Source: CAD feature listing. Evaluate the final solid. Frame: model axes, mm. A direction names the side the tool comes from. Give positions to 0.01 mm unless a question says otherwise; leave off trailing zeros. Write each loop counter-clockwise with the first axis right and the second up, starting at its lowest first coordinate (ties: lowest second). Pieces come first, ordered by that corner, then holes. Notation, with made-up numbers: (-5, 36) -> (27, 36) arc R19 ccw to (27, 69) -> close; hole circle Ø7 at (0.25, -13.5). An arc over 180 degrees is marked (long way). Answer as a JSON object with one key per item and string values. Group by question number.
Item 1: Pull-direction query (Y, two-part tool) for faces 4 (the face through (2, -1, 46.038)), 5 (the face through (2, 69.85, 25)), 6 (the face through (-127, -0.3, 27.4)); classes: pulls with the +Y half, pulls with the -Y half, needs draft (parallel to the pull), parting line crosses it, or undercut.
Item 2: Section query C-C on x = 106.5. Return the cut outline in (y, z), plus the area to 3 significant figures.
Item 3: Section query B-B on y = 11. Return the cut outline in (x, z), plus the area to 3 significant figures.
Item 4: Access query for faces 1 (the face through (2, 35, 0)), 2 (the face through (2, 0.127, 23)), 3 (the face through (2, 35, 4.762)). Directions: +Z, -Z, +X, -X, +Y, -Y. A direction counts if a zero-diameter tool reaches every point of the face in a straight line with its end or side. Return the directions, or none.
Item 5: Section query A-A on z = 9. Return the cut outline in (x, y).
Item 6: Ray query, probe 1 along Y at (x, z) = (20, 33); probe 2 along Z at (x, y) = (-25, 44); probe 3 along Y at (x, z) = (-112, 46). Return the intervals inside material, ascending. Write a range as from..to.
from build123d import *

# Parameters (mm, degrees)
F1_DEPTH = 127


with BuildPart() as f1:
    # F0 (on Right) → F1 (new body, symmetric)
    with BuildSketch(Plane.YZ):
        Polygon((69.85, 50.8), (-69.85, 50.8), (-69.85, 0), (-0.127, 0), (-0.127, 45.7835), (-4.7625, 45.7835), (-4.7625, 4.7625), (-65.0875, 4.7625), (-65.0875, 46.0375), (65.0875, 46.0375), (65.0875, 4.7625), (4.7625, 4.7625), (4.7625, 45.7835), (0.127, 45.7835), (0.127, 0), (69.85, 0), align=None)
    extrude(amount=F1_DEPTH, both=True)


solid = f1.part
Worked answers:
{
 "1": {"face 4": "undercut", "face 5": "pulls with the +Y half", "face 6": "needs draft"},
 "2": {"outline": "(-69.85, 0) -> (-0.13, 0) -> (-0.13, 45.78) -> (-4.76, 45.78) -> (-4.76, 4.76) -> (-65.09, 4.76) -> (-65.09, 46.04) -> (65.09, 46.04) -> (65.09, 4.76) -> (4.76, 4.76) -> (4.76, 45.78) -> (0.13, 45.78) -> (0.13, 0) -> (69.85, 0) -> (69.85, 50.8) -> (-69.85, 50.8) -> close", "area": "2,100 mm^2"},
 "3": {"outline": "(-127, 0) -> (127, 0) -> (127, 4.76) -> (-127, 4.76) -> close; (-127, 46.04) -> (127, 46.04) -> (127, 50.8) -> (-127, 50.8) -> close", "area": "2,420 mm^2"},
 "4": {"face 1": "-Z, +X, -X, +Y, -Y", "face 2": "-Z, +X, -X", "face 3": "+X, -X"},
 "5": {"outline": "(-127, -69.85) -> (127, -69.85) -> (127, -65.09) -> (-127, -65.09) -> close; (-127, -4.76) -> (127, -4.76) -> (127, -0.13) -> (-127, -0.13) -> close; (-127, 0.13) -> (127, 0.13) -> (127, 4.76) -> (-127, 4.76) -> close; (-127, 65.09) -> (127, 65.09) -> (127, 69.85) -> (-127, 69.85) -> close"},
 "6": {"probe 1": "-69.85..-65.09, -4.76..-0.13, 0.13..4.76, 65.09..69.85", "probe 2": "0..4.76, 46.04..50.8", "probe 3": "-69.85..-65.09, 65.09..69.85"}
}
